Source: CAD feature listing. Evaluate the final solid. Frame: model axes, mm. Face numbers are marked on the shaded views. A direction names the side the tool comes from. Coordinates: 2 decimals unless noted, no trailing zeros. Loops run counter-clockwise (first coordinate to the right, second up) from the corner with the lowest first, then second, coordinate; pieces in that order, holes last. Notation, with made-up numbers: (-9, -30.5) -> (14, -30.5) arc R17 ccw to (14, -4.5) -> close; hole circle Ø5 at (80.25, 87.25). An arc over 180 degrees is marked (long way). Answer as CSV lines item,"result".
from build123d import *


with BuildPart() as part:
    # Sketch1 → Revolve1 (revolve)
    with BuildSketch(Plane.XY, mode=Mode.PRIVATE) as revolve1_sk:
        with BuildLine():
            Line((6.635, 15.0004), (6, 15.0004))
            Line((6, 15.0004), (6, -15.0004))
            Line((6, -15.0004), (6.635, -15.0004))
            Line((6.635, -15.0004), (6.635, -14.594))
            ThreePointArc((6.635, -14.594), (6.709394878, -14.414394878), (6.889, -14.34))
            Line((6.889, -14.34), (9.435, -14.34))
            Line((9.435, -14.34), (9.435, -14.92))
            Line((9.435, -14.92), (9.977, -14.92))
            ThreePointArc((9.977, -14.92), (10.336210245, -14.771210245), (10.485, -14.412))
            Line((10.485, -14.412), (10.485, -11.325))
            Line((10.485, -11.325), (10, -11.325))
            Line((10, -11.325), (10, -10.125))
            Line((10, -10.125), (10.485, -10.125))
            Line((10.485, -10.125), (10.485, 10.125))
            Line((10.485, 10.125), (10, 10.125))
            Line((10, 10.125), (10, 11.325))
            Line((10, 11.325), (10.485, 11.325))
            Line((10.485, 11.325), (10.485, 14.412))
            ThreePointArc((10.485, 14.412), (10.336210245, 14.771210245), (9.977, 14.92))
            Line((9.977, 14.92), (9.435, 14.92))
            Line((9.435, 14.92), (9.435, 14.34))
            Line((9.435, 14.34), (6.889, 14.34))
            ThreePointArc((6.889, 14.34), (6.709394878, 14.414394878), (6.635, 14.594))
            Line((6.635, 14.594), (6.635, 15.0004))
        make_face()
    revolve(revolve1_sk.sketch.rotate(Axis((0, 15.0004, 0), (0, -1, 0)), 270), axis=Axis((0, 15.0004, 0), (0, -1, 0)))


solid = part.part
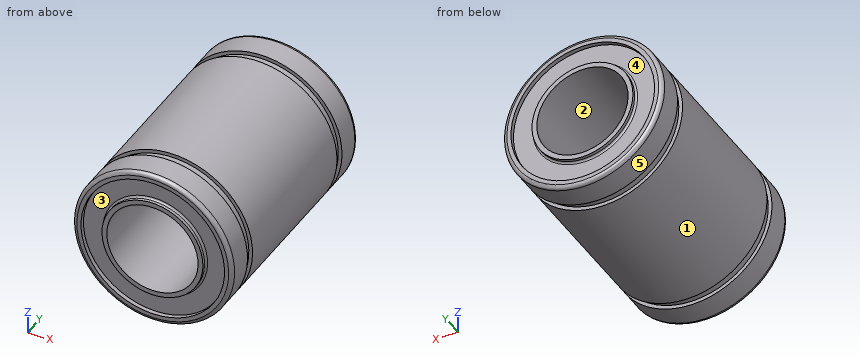
(1) Material intervals for L1, parallel to Y at x = 2.5, z = -7; L2, parallel to X at y = 14.75, z = 0 (3 decimals); L3, parallel to X at y = 1.5, z = 2, sorted ascending. Write a range as [from, to].
Computed values:
L1,"[-14.34, 14.34]"
L2,"[-10.356, -9.435], [-6.635, -6], [6, 6.635], [9.435, 10.356]"
L3,"[-10.29, -5.66], [5.66, 10.29]"
(2) Draft query along Z for the marked faces 1, 2 and 3. Return one class per face: released by +Z, released by -Z, zero draft, split by the parting line, or undercut.
Computed values:
face 1,"split by the parting line"
face 2,"undercut"
face 3,"undercut"
(3) Cut plane A-A (y = -8). Return the cut outline in (x, z) (3 decimals), then the cut area to 3 significant figures.
Computed values:
outline,"circle Ø20.97 at (0, 0); hole circle Ø12 at (0, 0)"
area,"232 mm^2"
(4) Access query for the marked faces 4 and 5. Directions: +Z, -Z, +X, -X, +Y, -Y. A direction counts if a zero-diameter tool reaches every point of the face in a straight line with its end or side. Return the directions, or none.
Computed values:
face 4,"+Y"
face 5,"+Y, -Y"
(5) Pin query (flat end, axial travel): pin 1 Ø4 at (x, y) = (5, 6.5) entering from +Z; pin 2 Ø2 at (x, y) = (-1.5, 1.5) entering from -Z; pin 3 Ø4 at (x, y) = (7.5, -10.5) entering from -Z. Return the tip coordinate at first contact, or that it passes through.
Computed values:
pin 1,"z = 10.05"
pin 2,"z = -10.47"
pin 3,"z = -8.9"
